Check sheet for the modelled part. Datum: model origin and axes. Units: mm. Face numbers are marked on the shaded views. A direction names the side the tool comes from. Round coordinates to 2 decimals unless told otherwise and drop trailing zeros. Write each loop counter-clockwise with the first axis right and the second up, starting at its lowest first coordinate (ties: lowest second). Pieces come first, ordered by that corner, then holes. Notation, with made-up numbers: (41, -14.5) -> (70, -14.5) arc R34 cw to (70, 22.5) -> close; hole circle Ø1 at (-14, -24). An arc over 180 degrees is marked (long way). Answer as a JSON object with one key per item and string values. Group by question number.
```python
from build123d import *

# Parameters (mm, degrees)
F0_W     = 76.2
F0_H     = 101.6
F1_DEPTH = 19.05
F2_W     = 63.5
F2_H     = 6.35
F3_DEPTH = 164.846


with BuildPart() as f1:
    # F0 (on Top) → F1 (new body)
    with BuildSketch(Plane.XY):
        Rectangle(F0_W, F0_H)
        with BuildLine():
            ThreePointArc((-38.1, 50.8), (-88.9, 0), (-38.1, -50.8))
            Line((-38.1, -50.8), (-38.1, 50.8))
        make_face()
    extrude(amount=F1_DEPTH)

    # F2 (on face) → F3 (cut)
    with BuildSketch(Plane.XZ.offset(50.8)):
        with Locations((-6.35, 3.175)):
            Rectangle(F2_W, F2_H)
        Polygon((25.4, -12.1961906552), (25.4, 0), (-38.1, 0), (-38.1, 6.35), (-98.2422232628, 6.35), (-98.2422232628, -12.1961906552), align=None)
    extrude(amount=-F3_DEPTH, mode=Mode.SUBTRACT)


solid = f1.part
```
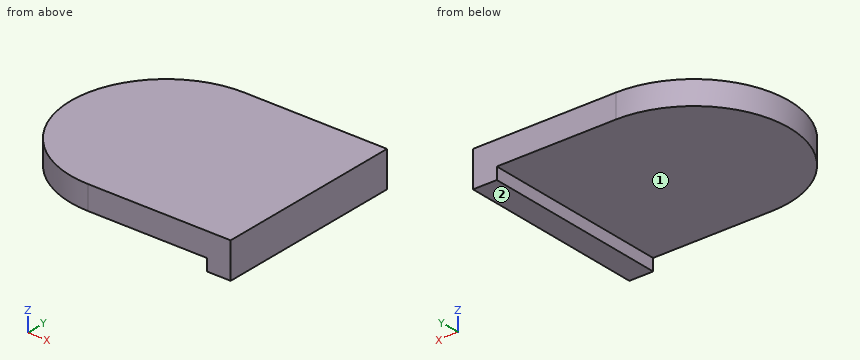
(1) Go/stop test with flat-tipped pins: pin 1 Ø7 at (y, z) = (19.5, 3.5) entering from -X; pin 2 Ø10 at (x, y) = (-27, -36) entering from -Z; pin 3 Ø4 at (x, z) = (-67, 5) entering from +Y. Record where each tip stops, or that it passes through.
(2) Section check C-C on z = 10. Record the cut outline in (x, y).
(3) Access from +Z, -Z, +X, -X, +Y, -Y to the whole of each face (thin tool, end or side, straight path). Record for the marked faces 1 and 2.
(4) Section check D-D on y = 0. Record the cut outline in (x, z), then the cut area to 3 significant figures.
(5) Scan lines: line 1 along Z through (x, y) = (-66.5, -23); line 2 along X through (y, z) = (5, 3); line 3 along X through (y, z) = (0.5, 15.75). Record each from-to range of solid material in increasing order.
(6) Section check A-A on y = 37. Record the cut outline in (x, z), then the cut area to 3 significant figures.
(7) Section check B-B on x = 3. Record the cut outline in (y, z), then the cut area to 3 significant figures.
Data:
{
 "1": {"pin 1": "stops at x = -85.8", "pin 2": "stops at z = 6.35", "pin 3": "stops at y = 42.76"},
 "2": {"outline": "(-38.1, -50.8) -> (38.1, -50.8) -> (38.1, 50.8) -> (-38.1, 50.8) arc R50.8 ccw to start"},
 "3": {"face 1": "-Z, -X, +Y, -Y", "face 2": "-Z, +X, -X, +Y, -Y"},
 "4": {"outline": "(-88.9, 6.35) -> (25.4, 6.35) -> (25.4, 0) -> (38.1, 0) -> (38.1, 19.05) -> (-88.9, 19.05) -> close", "area": "1,690 mm²"},
 "5": {"line 1": "z = 6.35 to 19.05", "line 2": "x = 25.4 to 38.1", "line 3": "x = -88.9 to 38.1"},
 "6": {"outline": "(-72.91, 6.35) -> (25.4, 6.35) -> (25.4, 0) -> (38.1, 0) -> (38.1, 19.05) -> (-72.91, 19.05) -> close", "area": "1,490 mm²"},
 "7": {"outline": "(-50.8, 6.35) -> (50.8, 6.35) -> (50.8, 19.05) -> (-50.8, 19.05) -> close", "area": "1,290 mm²"}
}
